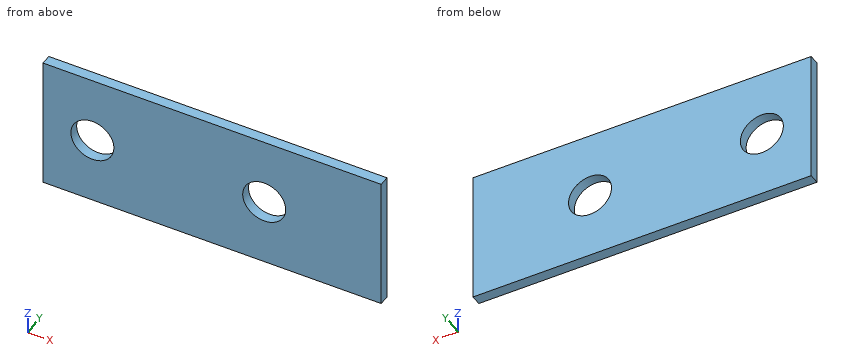
from build123d import *

# Parameters (mm, degrees)
SKETCH1_W           = 20
SKETCH1_H           = 10
SKETCH1_R           = 1.59
SKETCH1_W_2         = 5
BOSS_EXTRUDE1_DEPTH = 0.762


with BuildPart() as part:
    # Sketch1 → Boss-Extrude1 (new body)
    # profile 1 of 2: a face of its own
    with BuildSketch(Plane(origin=(0, 0, 0), x_dir=(1, 0, 0), z_dir=(0, 1, 0))):
        with Locations((6.35, 0)):
            Rectangle(SKETCH1_W, SKETCH1_H)
        with Locations(Location((0, 0, 0), (0, 0, 90))):
            Circle(SKETCH1_R, mode=Mode.SUBTRACT)
        with Locations(Location((12.7, 0, 0), (0, 0, 90))):
            Circle(SKETCH1_R, mode=Mode.SUBTRACT)
    # profile 2 of 2: a face of its own
    with BuildSketch(Plane(origin=(0, 0, 0), x_dir=(1, 0, 0), z_dir=(0, 1, 0))):
        with Locations((18.85, 0)):
            Rectangle(SKETCH1_W_2, SKETCH1_H)
    extrude(amount=BOSS_EXTRUDE1_DEPTH)


solid = part.part
Input: part model. Units: mm. Frame: model coordinates. Give positions to 0.01 mm unless a question says otherwise; leave off trailing zeros. Order: outer loops, then holes, each group sorted by start corner. A loop starts at its lowest first (then second) coordinate and runs counter-clockwise, first axis right, second up. Notation, with made-up numbers: (43.5, 51.5) - (87.5, 51.5) arc R23 cw to (87.5, 79.5) - close; hole circle Ø6 at (-3.5, -16). An arc over 180 degrees is marked (long way). Write each question's results on one line, items separated by ' | '.
Item 1: Material intervals for line 1 along X through (y, z) = (0.2, 0); line 2 along X through (y, z) = (0.3, -1); line 3 along Z through (x, y) = (12.7, 0.55), sorted ascending.
A:
line 1: x = -3.65 to -1.59, 1.59 to 11.11, 14.29 to 21.35 | line 2: x = -3.65 to -1.24, 1.24 to 11.46, 13.94 to 21.35 | line 3: z = -5 to -1.59, 1.59 to 5
Item 2: Section D-D (z = 1). Return loops of the section in (x, y).
A:
outline: (-3.65, 0) - (-1.24, 0) - (-1.24, 0.76) - (-3.65, 0.76) - close; (1.24, 0) - (11.46, 0) - (11.46, 0.76) - (1.24, 0.76) - close; (13.94, 0) - (21.35, 0) - (21.35, 0.76) - (13.94, 0.76) - close
Item 3: Contact query for a flat-ended pin moving along its axis: pin 1 Ø1 at (x, z) = (19, -0.5) entering from -Y. Output: stop coordinate, or through.
A:
pin 1: stops at y = 0
Item 4: Section A-A (z = 0). Return loops of the section in (x, y).
A:
outline: (-3.65, 0) - (-1.59, 0) - (-1.59, 0.76) - (-3.65, 0.76) - close; (1.59, 0) - (11.11, 0) - (11.11, 0.76) - (1.59, 0.76) - close; (14.29, 0) - (21.35, 0) - (21.35, 0.76) - (14.29, 0.76) - close
Item 5: Section C-C (y = 0.55). Return loops of the section in (x, z).
A:
outline: (-3.65, -5) - (21.35, -5) - (21.35, 5) - (-3.65, 5) - close; hole circle Ø3.18 at (0, 0); hole circle Ø3.18 at (12.7, 0)
Item 6: Section B-B (x = 12.7). Return loops of the section in (y, z).
A:
outline: (0, -5) - (0.76, -5) - (0.76, -1.59) - (0, -1.59) - close; (0, 1.59) - (0.76, 1.59) - (0.76, 5) - (0, 5) - close
